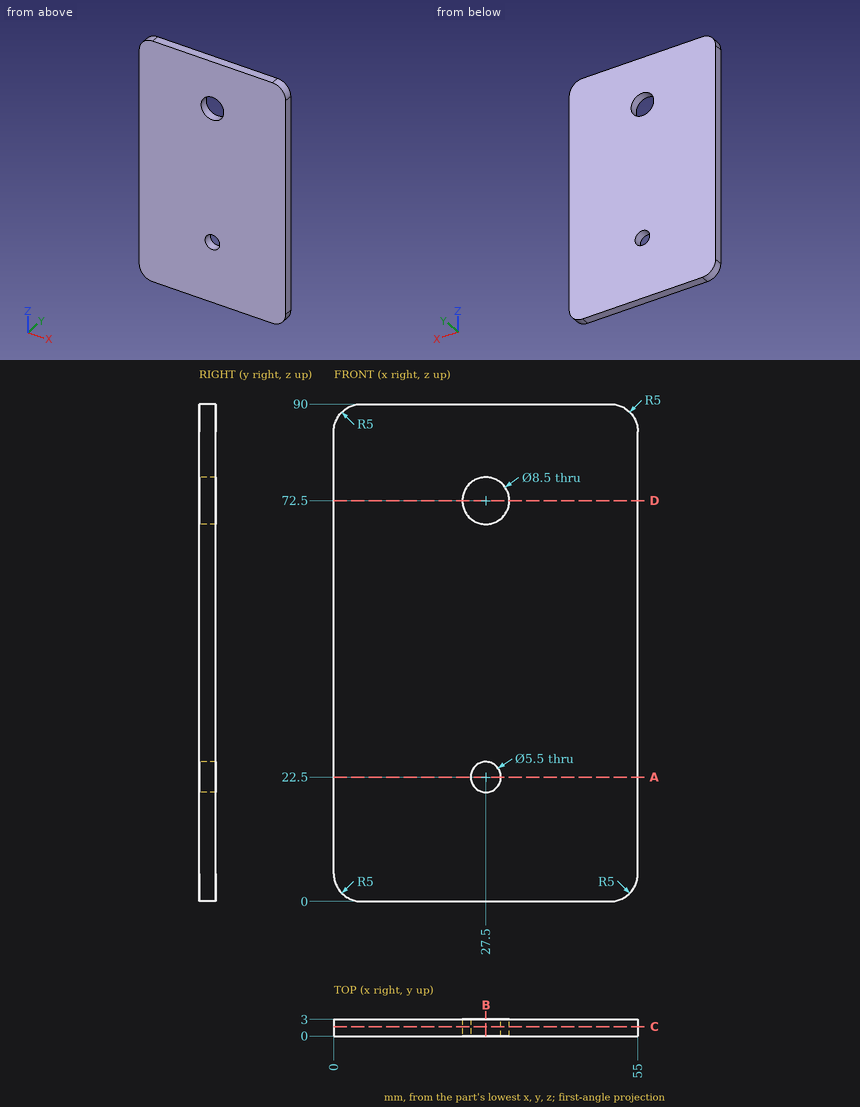
Geometry check sheet. Reference: drawing and pictorial views, mm from the part's lowest x, y, z. Coordinates: 2 decimals unless noted, no trailing zeros. Order: outer loops, then holes, each group sorted by start corner. A loop starts at its lowest first (then second) coordinate and runs counter-clockwise, first axis right, second up. Notation, with made-up numbers: (47, -37.75) -> (101, -37.75) arc R6 cw to (101, -28.75) -> close; hole circle Ø8 at (44, 72.25). An arc over 180 degrees is marked (long way). Use CSV: the item, a comma, the result in double quotes. Start each with the question number.
Q1. Section check A-A, the plane z = 22.5. Record the cut outline in (x, y), and give its area (4 significant figures).
Q2. Section check D-D, the plane z = 72.5. Record the cut outline in (x, y), and give its area (4 significant figures).
Q3. Thickness scan on line 1 along Z through (x, y) = (27.5, 1.55). Record the ranges inside material, lowest first.
Q4. Section check B-B, the plane x = 27.5. Record the cut outline in (y, z).
Q5. Section check C-C, the plane y = 1.7. Record the cut outline in (x, z), and give its area (3 significant figures).
Returned:
1,outline,"(0, 0) -> (24.75, 0) -> (24.75, 3) -> (0, 3) -> close; (30.25, 0) -> (55, 0) -> (55, 3) -> (30.25, 3) -> close"
1,area,"148.5 mm^2"
2,outline,"(0, 0) -> (23.25, 0) -> (23.25, 3) -> (0, 3) -> close; (31.75, 0) -> (55, 0) -> (55, 3) -> (31.75, 3) -> close"
2,area,"139.5 mm^2"
3,line 1,"z = 0 to 19.75, 25.25 to 68.25, 76.75 to 90"
4,outline,"(0, 0) -> (3, 0) -> (3, 19.75) -> (0, 19.75) -> close; (0, 25.25) -> (3, 25.25) -> (3, 68.25) -> (0, 68.25) -> close; (0, 76.75) -> (3, 76.75) -> (3, 90) -> (0, 90) -> close"
5,outline,"(0, 5) arc R5 ccw to (5, 0) -> (50, 0) arc R5 ccw to (55, 5) -> (55, 85) arc R5 ccw to (50, 90) -> (5, 90) arc R5 ccw to (0, 85) -> close; hole circle Ø8.5 at (27.5, 72.5); hole circle Ø5.5 at (27.5, 22.5)"
5,area,"4,850 mm^2"
